```python
from build123d import *

# Parameters (mm, degrees)
F3_DEPTH = 160.02


with BuildPart() as f1:
    # F0 (on Front) → F1 (revolve)
    with BuildSketch(Plane.XZ):
        Polygon((11.633136, 25.396974), (0, 50.8), (0, 0), (8.89, 0), (8.89, 20.170162), (57.288211, 35.605614), (57.288211, 86.405614), align=None)
    revolve(axis=Axis((0, 0, 25.4), (0, 0, -1)))

    # F2 (on Right) → F3 (cut)
    with BuildSketch(Plane.YZ):
        Polygon((0, 55.20786), (-18.9991, 74.483134), (-18.9991, 44.67614), (13.663266, 55.20786), align=None)
    extrude(amount=-F3_DEPTH, mode=Mode.SUBTRACT)


solid = f1.part
```
CAD build for the part. Positions are in the model's coordinates, mm. A direction names the side the tool comes from. Give positions to 0.01 mm unless a question says otherwise; leave off trailing zeros. Order: outer loops, then holes, each group sorted by start corner. A loop starts at its lowest first (then second) coordinate and runs counter-clockwise, first axis right, second up. Notation, with made-up numbers: M 38.25,58 L 48.25,58 A16 ccw 48.25,71 Z; hole C 85,-36.75 d5. An arc over 180 degrees is marked long. Put each result on its own line as item: value. Start each with the question number.
(1) Saw through at C-C, the plane z = 5. Write the cut outline in (x, y), then the cut area to 3 significant figures.
(2) Which spindle directions (+Z, -Z, +X, -X, +Y, -Y) get a long thin tool onto all of the face, cutting with end or side? Do faces 4 (the cylindrical face through (-1.93, 8.68, 10.23)), 5 (the conical face through (22.89, -7.21, 41.92)). Say none if no direction does.
(3) Saw through at A-A, the plane z = 49. Write the cut outline in (x, y), then the cut area to 3 significant figures.
(4) Drill centre lines: line 1 along Y through (x, z) = (-52, 60.5); line 2 along X through (y, z) = (-1.5, 58.5); line 3 along X through (y, z) = (14.5, 40.5). Where is each one in solid material? Low to high.
(5) Saw through at D-D, the plane z = 29. Write the cut outline in (x, y), then the cut area to 3 significant figures.
(6) Flat gauge pins, fed straight in: pin 1 Ø1.5 at (x, y) = (44, 7) entering from +Z; pin 2 Ø12 at (y, z) = (-34.5, 36) entering from -X; pin 3 Ø1 at (x, y) = (-7.5, -9) entering from +Z. Where does each tip first touch, or does it go through?
(7) Mould opens along Y. For faces 1 (the flat face through (-48.046, -7.256, 62.569)), 2 (the flat face through (0, 0, 0)), 3 (the cylindrical face through (54.64, -17.21, 61.36)) say: +Y half, -Y half, draft (parallel to the pull), parting line (faces both ways), or undercut.
(8) Saw through at B-B, the plane z = 79. Write the cut outline in (x, y).
Check result:
1. outline: C 0,0 d17.78
1. area: 248 mm2
2. face 4: -Z
2. face 5: +Z
3. outline: M -57.01,-5.59 L -28.76,-5.59 A29.3 cw long -22.3,-19 L -54.05,-19 A57.29 ccw long Z; C 0,0 d1.65
3. area: 7,220 mm2
4. line 1: y = -24.04 to -19, -5.22 to 24.04
4. line 2: x = -57.27 to -36.37, 36.37 to 57.27
4. line 3: x = -55.42 to -17.77, 17.77 to 55.42
5. outline: C 0,0 d73.15; C 0,0 d19.97; hole C 0,0 d28.66
5. area: 3,870 mm2
6. pin 1: stops at z = 70.39
6. pin 2: stops at x = -49.7
6. pin 3: stops at z = 26.31
7. face 1: undercut
7. face 2: draft
7. face 3: parting line
8. outline: C 0,0 d114.58; hole C 0,0 d103.49
